```python
from build123d import *

# Parameters (mm, degrees)
EXTRUDE1_REACH           = 60.029
LPATTERN1_COUNT          = 38
LPATTERN1_PITCH          = 1.25
SKETCH11_W               = 5.6
SKETCH11_H               = 0.666666667
POINT_CUT_EXTRUDE8_DEPTH = 52.391828144
SKETCH16_R               = 4
CUT_EXTRUDE1_DEPTH       = 1.12


with BuildPart() as part:
    # Sketch1 → base-Revolve (revolve)
    with BuildSketch(Plane.XY, mode=Mode.PRIVATE) as base_revolve_sk:
        with BuildLine():
            Line((0, 8.4), (-1.2, 8.4))
            Line((-1.2, 8.4), (-2.304726967, 5))
            Line((-2.304726967, 5), (-6.8, 5))
            Line((-6.8, 5), (-6.8, 0))
            Line((-6.8, 0), (-5.68, 0))
            Line((-5.68, 0), (0, 0))
            Line((0, 0), (50, 0))
            Line((50, 0), (50, 4))
            Line((50, 4), (2.5, 4))
            Line((2.5, 4), (1.7, 3.2))
            Line((1.7, 3.2), (0.5, 3.2))
            ThreePointArc((0.5, 3.2), (0.146446609, 3.346446609), (0, 3.7))
            Line((0, 3.7), (0, 8.4))
        make_face()
    revolve(base_revolve_sk.sketch.rotate(Axis((0, 0, 0), (1, 0, 0)), 90), axis=Axis((0, 0, 0), (1, 0, 0)))

    # Extrude1: up to this cone (the profile starts outside it)
    extrude1_end = Plane(origin=(-6.8, 0, 0), z_dir=(1, 0, 0)).offset(2.870675552) * Cone(3.078e-06, 177.454079013, 57.658324448, align=(Align.CENTER, Align.CENTER, Align.MIN), mode=Mode.PRIVATE)
    # Sketch15 → Extrude1 (add, up to the surface)
    with BuildSketch(Plane.ZY.offset(6.8), mode=Mode.PRIVATE) as extrude1_sk1:
        Polygon((-2.886751346, 5), (-5.773502692, 0), (-2.886751346, -5), (2.886751346, -5), (5.773502692, 0), (2.886751346, 5), align=None)
    extrude1_tool1 = extrude(extrude1_sk1.sketch, amount=-EXTRUDE1_REACH, mode=Mode.PRIVATE) - extrude1_end
    add(extrude1_tool1.solids().sort_by_distance((-6.8, 0, 0))[0])

    # thd_Sketch7 → thd_Cut-Revolve2 (revolve, cut)
    with BuildSketch(Plane.XY, mode=Mode.PRIVATE) as thd_cut_revolve2_sk:
        Polygon((2.038119785, 4.923760431), (2.038119785, 4), (2.5, 3.2), (2.826239569, 3.2), (3.288119785, 4), (3.288119785, 4.923760431), (2.961880215, 4.923760431), align=None)
    thd_cut_revolve2 = revolve(thd_cut_revolve2_sk.sketch.rotate(Axis((0, 0, 0), (1, 0, 0)), 90), axis=Axis((0, 0, 0), (1, 0, 0)), mode=Mode.SUBTRACT)

    # LPattern1: thd_Cut-Revolve2 ×38
    with Locations(*[(i * LPATTERN1_PITCH, 0, 0) for i in range(1, LPATTERN1_COUNT)]):
        add(thd_cut_revolve2, mode=Mode.SUBTRACT)

    # Sketch8 → point_Cut-Revolve1 (revolve, cut)
    with BuildSketch(Plane.XY, mode=Mode.PRIVATE) as point_cut_revolve1_sk:
        Polygon((50, 0), (50.508, 0), (50.508, 4.508), (48.614359354, 4.508), (48.614359354, 4), (50, 3.2), align=None)
    revolve(point_cut_revolve1_sk.sketch.rotate(Axis((0, 0, 0), (1, 0, 0)), 90), axis=Axis((0, 0, 0), (1, 0, 0)), mode=Mode.SUBTRACT)

    # Sketch11 → point_Cut-Extrude8 (cut, through all)
    with BuildSketch(Plane.XY):
        with Locations((47.2, -0.333333333)):
            Rectangle(SKETCH11_W, SKETCH11_H)
    extrude(amount=POINT_CUT_EXTRUDE8_DEPTH, mode=Mode.SUBTRACT)

    # Sketch16 → Cut-Extrude1 (cut)
    with BuildSketch(Plane.ZY.offset(6.8)):
        Circle(SKETCH16_R)
    extrude(amount=-CUT_EXTRUDE1_DEPTH, mode=Mode.SUBTRACT)


solid = part.part
```
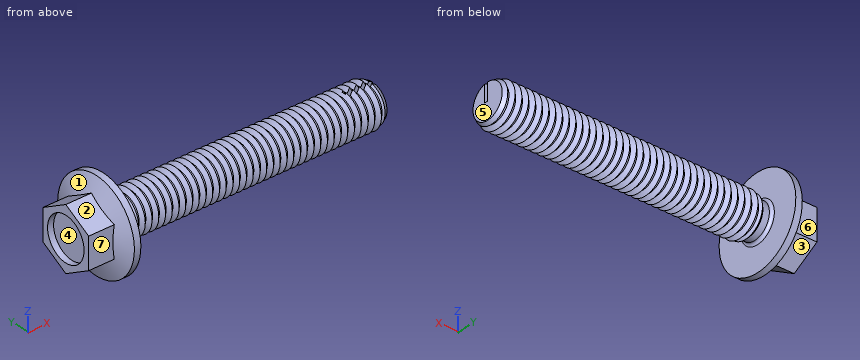
The listing builds one solid part. Answer for the finished solid, in the listing's coordinates (mm). Face numbers are marked on the shaded views. A direction names the side the tool comes from. Give positions to 0.01 mm unless a question says otherwise; leave off trailing zeros. One line per item, written item: value.
1. For a pull along Y with two mould halves and no side action, classify the marked faces 4, 5, 6 and 7 as pulls with the +Y half, pulls with the -Y half, needs draft (parallel to the pull), parting line crosses it, or undercut.
Found:
face 4: undercut
face 5: needs draft
face 6: pulls with the +Y half
face 7: pulls with the -Y half
2. For the marked faces 1, 2 and 3, determine the directions among +Z, -Z, +X, -X, +Y, -Y from which every point of the face is accessible in a straight line to the end or side of a thin tool.
Found:
face 1: -X
face 2: +Z, -X, -Y
face 3: -Z, -X, +Y
3. Find the intervals of material crossed by probe 1 along Y at (x, z) = (-6.5, 0); probe 2 along X at (y, z) = (-4, 3); probe 3 along X at (y, z) = (-2.5, -0.75), in increasing order.
Found:
probe 1: -5 to -4, 4 to 5
probe 2: -6.8 to 0
probe 3: -5.68 to 50
4. Each of these flat-tipped pins is pushed along its axis until it touches: P1, Ø6.5, axis at y = 1, z = -1, coming from the -X side; P2, Ø1.5, axis at x = 24, z = -6, coming from the +Y side; P3, Ø10, axis at x = 36, z = 5, coming from the +Y side; P4, Ø4, axis at x = 20.5, z = -1, coming from the -Y side. Where does it stop, or does it pass through?
Found:
P1: x = -6.8
P2: through
P3: y = 4
P4: y = -4
